Design review of the part shown in the three views and the two pictorial views. Dimensions are in mm from the part's minimum x, y and z. A direction names the side the tool comes from. Round coordinates to 2 decimals unless told otherwise and drop trailing zeros. One line per question, with ' | ' between items. Start each with the question number.
1) Mouldability with a two-part tool opening along Z and no side actions: class the marked faces 1, 2, 3 and 4 as +Z half, -Z half, draft (parallel to the pull), parting line (faces both ways), or undercut.
2) Insertion check: pin 1 Ø9.5 at (x, y) = (55, 19.5) entering from -Z. The pin has a flat end and moves straight along its axis. Give the tip position at first contact, or say it passes through.
3) Consider section A-A (x = 77.5). Count the separate pieces of the cut face and the enclosed holes in it.
4) For probe 1 along Z at (x, y) = (13, 28); probe 2 along X at (y, z) = (11, 18.5) (1 decimal); probe 3 along X at (y, z) = (6, 152.5), list the stretches that pass through material, from the lowest coordinate up.
5) For the marked faces 5 and 6, list the 3-axis set-ups (+Z, -Z, +X, -X, +Y, -Y) from which the entire face can be reached by the end or side of a thin tool; tool diameter is ignored.
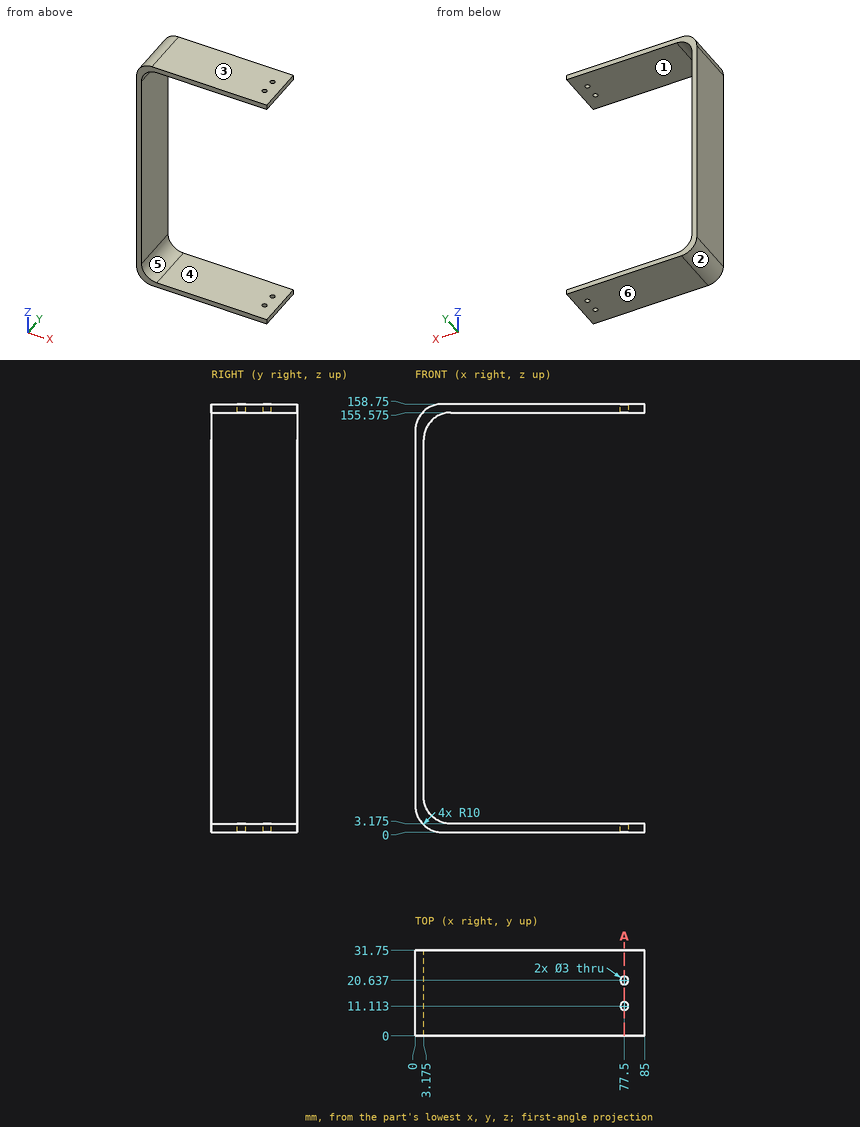
From the geometry:
1) face 1: undercut | face 2: -Z half | face 3: +Z half | face 4: undercut
2) pin 1: stops at z = 0
3) separate pieces: 6 | enclosed holes: 0
4) probe 1: z = 0 to 3.18, 155.57 to 158.75 | probe 2: x = 0 to 3.2 | probe 3: x = 0.73 to 5.96
5) face 5: +X, +Y, -Y | face 6: -Z, +X, -X, +Y, -Y
